Verification items for the finished model (mm, model axes). Face numbers are marked on the shaded views. A direction names the side the tool comes from. Round coordinates to 2 decimals unless told otherwise and drop trailing zeros. Write each loop counter-clockwise with the first axis right and the second up, starting at its lowest first coordinate (ties: lowest second). Pieces come first, ordered by that corner, then holes. Notation, with made-up numbers: M 86.5,34 L 120.5,34 A5 cw 120.5,42 Z; hole C 44,45.5 d1. An arc over 180 degrees is marked long. Use a Markdown table: item, result. Add a question column.
from build123d import *

# Parameters (mm, degrees)
SKETCH_W        = 20
SKETCH_H        = 47.4
PAD_DEPTH       = 12.5
POCKET_DEPTH    = 12.501
POCKET001_DEPTH = 47.401
SKETCH003_W     = 20
SKETCH003_H     = 8
POCKET002_DEPTH = 9
SKETCH004_W     = 28
SKETCH004_H     = 8.15
POCKET003_DEPTH = 3.751
SKETCH005_W     = 27.5
SKETCH005_H     = 1
PAD001_DEPTH    = 5
SKETCH006_W     = 24
SKETCH006_H     = 5.5
PAD002_DEPTH    = 4.8
FILLET_R        = 2.5
FILLET001_R     = 3
POCKET004_DEPTH = 3.501


with BuildPart() as part:
    # Sketch → Pad (new body)
    with BuildSketch(Plane.YZ):
        with Locations((-2.5, 0)):
            Rectangle(SKETCH_W, SKETCH_H)
    extrude(amount=PAD_DEPTH)

    # Sketch001 (on Face6 of Pad) → Pocket (cut, through all)
    with BuildSketch(Plane.YZ.offset(12.5)):
        with BuildLine():
            Line((-7.5, 23.7), (-7.5, 15.75))
            ThreePointArc((-7.5, 15.75), (-11.25, 0), (-7.5, -15.75))
            Line((-7.5, -15.75), (-7.5, -23.7))
            Line((-7.5, -23.7), (-12.5, -23.7))
            Line((-12.5, -23.7), (-12.5, 23.7))
            Line((-12.5, 23.7), (-7.5, 23.7))
        make_face()
    extrude(amount=-POCKET_DEPTH, mode=Mode.SUBTRACT)

    # Sketch002 (on Face6 of Pocket) → Pocket001 (cut, through all)
    with BuildSketch(Plane.YX.offset(23.7)):
        Polygon((7.5, 0), (7.5, 12.5), (5.5, 12.5), align=None)
    extrude(amount=-POCKET001_DEPTH, mode=Mode.SUBTRACT)

    # Sketch003 (on Face4 of Pocket001) → Pocket002 (cut)
    with BuildSketch(Plane.YZ.offset(12.5)):
        with Locations((-2.5, 19.7)):
            Rectangle(SKETCH003_W, SKETCH003_H)
        with Locations((-2.5, -19.7)):
            Rectangle(SKETCH003_W, SKETCH003_H)
    extrude(amount=-POCKET002_DEPTH, mode=Mode.SUBTRACT)

    # Sketch004 (on Face3 of Pocket002) → Pocket003 (cut, through all)
    with BuildSketch(Plane(origin=(0, -7.5, 0), x_dir=(0, 0, -1), z_dir=(0, -1, 0))):
        with Locations((0, 7.075)):
            Rectangle(SKETCH004_W, SKETCH004_H)
    extrude(amount=POCKET003_DEPTH, mode=Mode.SUBTRACT)

    # Sketch005 (on Face17 of Pocket003) → Pad001 (join)
    with BuildSketch(Plane(origin=(0, -7.5, 0), x_dir=(0, 0, -1), z_dir=(0, -1, 0))):
        with Locations((0, 10.25)):
            Rectangle(SKETCH005_W, SKETCH005_H)
        with Locations((0, 3.75)):
            Rectangle(SKETCH005_W, SKETCH005_H)
    extrude(amount=PAD001_DEPTH)

    # Sketch006 (on Face17 of Pad001) → Pad002 (join)
    with BuildSketch(Plane(origin=(0, -7.5, 0), x_dir=(0, 0, -1), z_dir=(0, -1, 0))):
        with Locations((0, 7)):
            Rectangle(SKETCH006_W, SKETCH006_H)
    extrude(amount=PAD002_DEPTH)

    # Fillet
    fillet_edges = [part.edges().sort_by_distance(p)[0] for p in [
        (10.25, -12.5, 13.75),
        (3.75, -12.5, 13.75),
        (10.25, -12.5, -13.75),
        (3.75, -12.5, -13.75),
    ]]
    fillet(fillet_edges, radius=FILLET_R)

    # Fillet001
    fillet001_edges = [part.edges().sort_by_distance(p)[0] for p in [
        (1.75, -7.5, 23.7),
        (1.75, 7.22, 23.7),
        (1.75, 7.22, -23.7),
        (1.75, -7.5, -23.7),
    ]]
    fillet(fillet001_edges, radius=FILLET001_R)

    # Sketch007 (on Face12 of Fillet001) → Pocket004 (cut, through all)
    with BuildSketch(Plane.YZ.offset(3.5)):
        with BuildLine():
            ThreePointArc((-2.9, 21.8), (-4.7, 20), (-2.9, 18.2))
            Line((-2.9, 18.2), (2.9, 18.2))
            ThreePointArc((2.9, 18.2), (4.7, 20), (2.9, 21.8))
            Line((-2.9, 21.8), (2.9, 21.8))
        make_face()
        with BuildLine():
            ThreePointArc((-2.9, -18.2), (-4.7, -20), (-2.9, -21.8))
            Line((-2.9, -21.8), (2.9, -21.8))
            ThreePointArc((2.9, -21.8), (4.7, -20), (2.9, -18.2))
            Line((-2.9, -18.2), (2.9, -18.2))
        make_face()
    extrude(amount=-POCKET004_DEPTH, mode=Mode.SUBTRACT)


solid = part.part
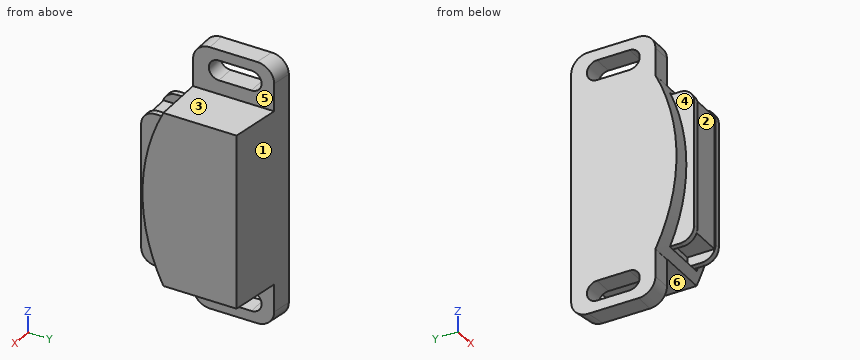
1. Cross-section at B-B on y = -10.5. Enter the section's corners in (x, z), plus the area to 3 significant figures.
2. Cross-section at D-D on z = -6. Enter the section's corners in (x, y), plus the area to 3 significant figures.
3. Cross-section at C-C on z = 4. Enter the section's corners in (x, y), plus the area to 3 significant figures.
4. Access from +Z, -Z, +X, -X, +Y, -Y to the whole of each face (thin tool, end or side, straight path). Record for the marked faces 1, 2 and 3.
5. Depth check by flat-ended pin: pin 1 Ø6 at (x, z) = (10, -7.5) entering from +Y; pin 2 Ø5.5 at (x, y) = (7, -9) entering from -Z; pin 3 Ø2 at (x, z) = (6, -12.5) entering from +Y. Enter the tip coordinate at first touch or a pass-through.
6. Scan lines: line 1 along X through (y, z) = (-9, -11); line 2 along Z through (x, y) = (2.75, -1.75); line 3 along Z through (x, y) = (2, -4.5). Record each from-to range of solid material in increasing order. Write a range as from..to.
7. Cross-section at A-A on z = 20. Enter the section's corners in (x, y).
8. Release check for a two-part mould opening along X. For the marked faces 4, 5 and 6 record: +X half, -X half, draft (parallel to the pull), parting line (faces both ways), or undercut.
Answer:
| question | item | result |
|---|---|---|
| 1 | outline | M 0,-7.2 L 3,-7.2 L 3,7.2 L 0,7.2 Z; M 3.25,-13.7 L 4.25,-13.7 L 4.25,-12 L 9.75,-12 L 9.75,-13.7 L 10.75,-13.7 L 10.75,13.7 L 9.75,13.7 L 9.75,12 L 4.25,12 L 4.25,13.7 L 3.25,13.7 Z; M 11.15,-7.2 L 12.5,-7.2 L 12.5,7.2 L 11.15,7.2 Z |
| 1 | area | 249 mm^2 |
| 2 | outline | M 0,-10.73 L 3,-10.73 L 3,-7.5 L 3.25,-7.5 L 3.25,-12.5 L 4.25,-12.5 L 4.25,-12.3 L 9.75,-12.3 L 9.75,-12.5 L 10.75,-12.5 L 10.75,-7.5 L 11.15,-7.5 L 11.15,-10.73 L 12.5,-10.73 L 12.5,5.5 L 0,7.5 Z |
| 2 | area | 225 mm^2 |
| 3 | outline | M 0,-11.02 L 3,-11.02 L 3,-7.5 L 3.25,-7.5 L 3.25,-12.5 L 4.25,-12.5 L 4.25,-12.3 L 9.75,-12.3 L 9.75,-12.5 L 10.75,-12.5 L 10.75,-7.5 L 11.15,-7.5 L 11.15,-11.02 L 12.5,-11.02 L 12.5,5.5 L 0,7.5 Z |
| 3 | area | 227 mm^2 |
| 4 | face 1 | +Z, -Z, +X, +Y |
| 4 | face 2 | +Z, -Z, -Y |
| 4 | face 3 | +Z, +X, +Y, -Y |
| 5 | pin 1 | stops at y = 6.38 |
| 5 | pin 2 | stops at z = -15.7 |
| 5 | pin 3 | stops at y = 6.7 |
| 6 | line 1 | x = 0..3, 3.25..10.75, 11.15..12.5 |
| 6 | line 2 | z = -23.7..-21.8, -18.2..18.2, 21.8..23.7 |
| 6 | line 3 | z = -23.7..-20.82, -19.18..19.18, 20.82..23.7 |
| 7 | outline | M 0,-7.5 L 3.5,-7.5 L 3.5,-4.7 L 0,-4.7 Z; M 0,4.7 L 3.5,4.7 L 3.5,6.94 L 0,7.5 Z |
| 8 | face 4 | undercut |
| 8 | face 5 | +X half |
| 8 | face 6 | draft |
